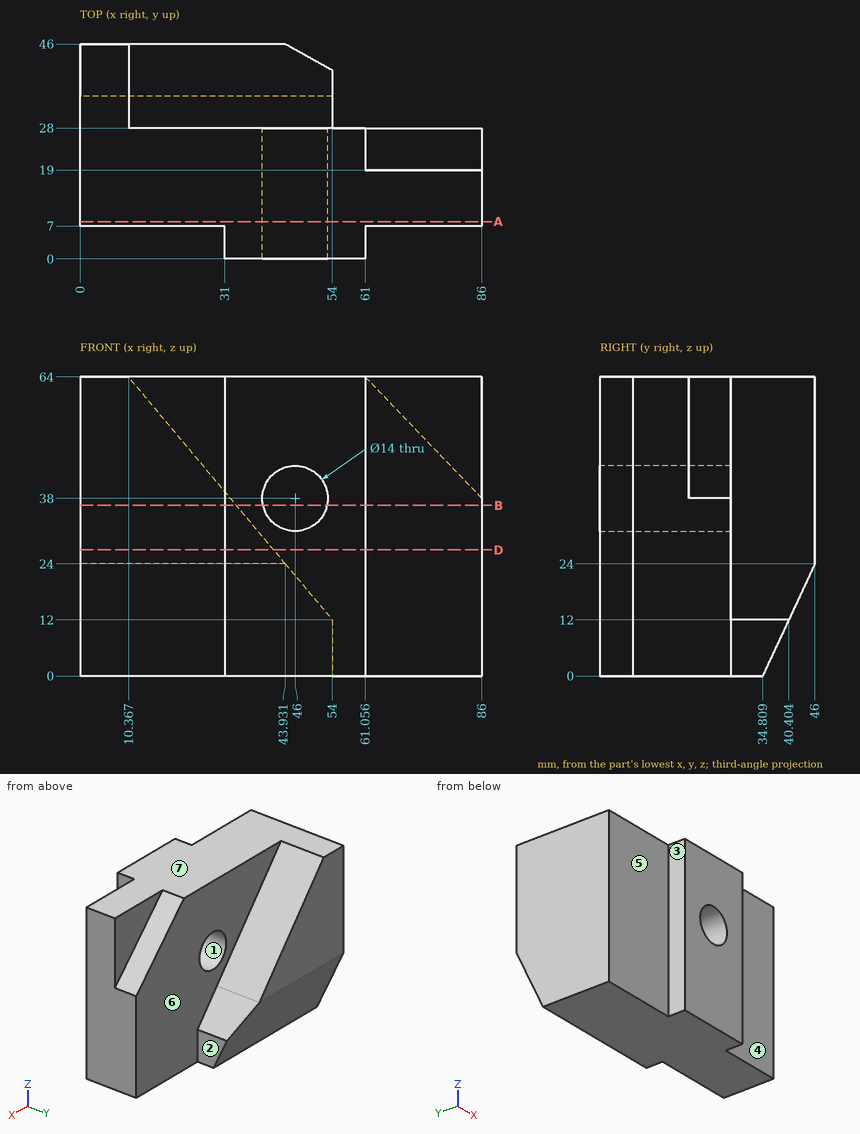
Can you work these out from the drawing? Everything is in mm from the part's minimum corner. A direction names the side the tool comes from. Coordinates: 2 decimals unless noted, no trailing zeros. Order: outer loops, then holes, each group sorted by start corner. A loop starts at its lowest first (then second) coordinate and runs counter-clockwise, first axis right, second up. Notation, with made-up numbers: (32, 89.25) -> (91, 89.25) arc R9 cw to (91, 98.25) -> close; hole circle Ø7 at (-36, 46.5). An arc over 180 degrees is marked (long way). Return JSON: item names as keys, results as strings.
1) On a 3-axis mill with a long thin cutter (end or side, diameter ignored), from which of +Z, -Z, +X, -X, +Y, -Y can I reach the whole of each face in a straight line? I mean the marked faces 4, 5, 6 and 7. Say none if no direction works.
Conclusion:
{"face 4": "+Z, -Z, +X, -Y", "face 5": "+Z, -Z, -X, -Y", "face 6": "+Z, +X, +Y", "face 7": "+Z, +X, -X, +Y, -Y"}
2) If we section it at D-D on z = 27: List the corners of the cut face in (x, y) for me, plus the area to 3 significant figures.
Conclusion:
{"outline": "(0, 7) -> (31, 7) -> (31, 0) -> (61, 0) -> (61, 7) -> (86, 7) -> (86, 28) -> (41.41, 28) -> (41.41, 46) -> (0, 46) -> close", "area": "2,760 mm²"}
3) If I drill on probe 1 along X at (y, z) = (16, 38); probe 2 along Y at (x, z) = (72.5, 52.5); probe 3 along Y at (x, z) = (32, 52), over which ranges is the centre line in solid material (lowest first)?
Conclusion:
{"probe 1": "x = 0 to 39, 53 to 86", "probe 2": "y = 7 to 19", "probe 3": "y = 0 to 28"}
4) Thinking about a two-plate mould opening in X: for the marked faces 1, 2 and 3, which applies, +X half, -X half, draft (parallel to the pull), parting line (faces both ways), or undercut?
Conclusion:
{"face 1": "undercut", "face 2": "+X half", "face 3": "-X half"}
5) If we section it at A-A on y = 8: List the corners of the cut face in (x, z) for me, plus the area to 3 significant figures.
Conclusion:
{"outline": "(0, 0) -> (86, 0) -> (86, 64) -> (0, 64) -> close; hole circle Ø14 at (46, 38)", "area": "5,350 mm²"}
6) If we section it at B-B on z = 36.5: List the corners of the cut face in (x, y) for me, plus the area to 4 significant figures.
Conclusion:
{"outline": "(0, 7) -> (31, 7) -> (31, 0) -> (39.16, 0) -> (39.16, 28) -> (33.44, 28) -> (33.44, 46) -> (0, 46) -> close; (52.84, 0) -> (61, 0) -> (61, 7) -> (86, 7) -> (86, 28) -> (52.84, 28) -> close", "area": "2,235 mm²"}
7) I'm going to push flat-ended pins straight in: P1, Ø3.5, axis at y = 3.5, z = 21.5, coming from the +X side; P2, Ø12.5, axis at x = 46, z = 38, coming from the +Y side; P3, Ø4, axis at x = 23.5, z = 31, coming from the -Y side; P4, Ø2, axis at x = 64, z = 38, coming from the +Y side. Where does each tip first touch, or does it pass through?
Conclusion:
{"P1": "stops at x = 61", "P2": "passes through", "P3": "stops at y = 7", "P4": "stops at y = 28"}
